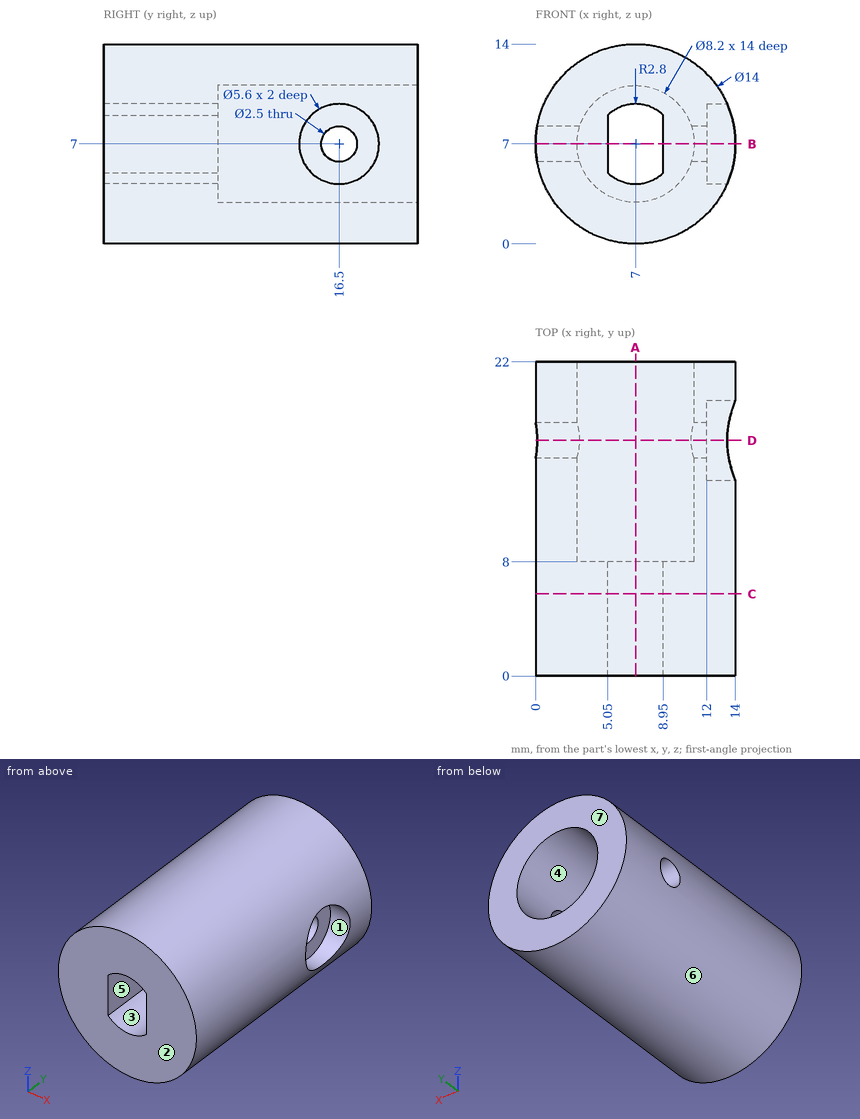
Drawing for the job (mm, zero at the part's lowest x, y, z). A direction names the side the tool comes from. Give positions to 0.01 mm unless a question says otherwise; leave off trailing zeros. Order: outer loops, then holes, each group sorted by start corner. A loop starts at its lowest first (then second) coordinate and runs counter-clockwise, first axis right, second up. Notation, with made-up numbers: (16, 34.25) - (41, 34.25) arc R21 cw to (41, 39.25) - close; hole circle Ø11 at (24.25, 49.25). An arc over 180 degrees is marked (long way). Use one line per item in the form item = value.
Item 1: Slice it at D-D on y = 16.5. Give the cut face in (x, z), and give its area (3 significant figures).
Solution:
outline = (0.11, 5.75) arc R7 ccw to (13.42, 4.2) - (12, 4.2) - (12, 5.75) - (10.9, 5.75) arc R4.1 cw to (3.1, 5.75) - close; (0.11, 8.25) - (3.1, 8.25) arc R4.1 cw to (10.9, 8.25) - (12, 8.25) - (12, 9.8) - (13.42, 9.8) arc R7 ccw to start
area = 81.3 mm2
Item 2: Pin check, flat tips, straight feed: pin 1 Ø3 at (y, z) = (16.5, 7) entering from -X; pin 2 Ø1.5 at (y, z) = (9, 2.5) entering from +X; pin 3 Ø5 at (y, z) = (16.5, 7) entering from +X; pin 4 Ø4 at (x, z) = (7.5, 6) entering from +Y. Stop position of each tip, or through.
Solution:
pin_1 = 0
pin_2 = 12.91
pin_3 = 12
pin_4 = 8
Item 3: Slice it at C-C on y = 5.75. Give the cut face in (x, z), and give its area (3 significant figures).
Solution:
outline = circle Ø14 at (7, 7); hole (5.05, 4.99) arc R2.8 ccw to (8.95, 4.99) - (8.95, 9.01) arc R2.8 ccw to (5.05, 9.01) - close
area = 134 mm2
Item 4: Which spindle directions (+Z, -Z, +X, -X, +Y, -Y) get a long thin tool onto all of the face, cutting with end or side? Do the marked faces 1, 2 and 3. Say none if no direction does.
Solution:
face_1 = +X
face_2 = +Z, -Z, +X, -X, -Y
face_3 = +Y, -Y
Item 5: Probe probe 1 along Y at (x, z) = (2.15, 7); probe 2 along Y at (x, z) = (12.5, 7); probe 3 along Y at (x, z) = (7.75, 10). List the from-to ranges inside material, lowest first. Write a range as from..to.
Solution:
probe_1 = 0..15.25, 17.75..22
probe_2 = 0..13.7, 19.3..22
probe_3 = 0..8
Item 6: Two-plate mould, pull along X, no slides. Class the marked faces 4, 5, 6 and 7: released by +X, released by -X, zero draft, split by the parting line, or undercut.
Solution:
face_4 = undercut
face_5 = undercut
face_6 = split by the parting line
face_7 = zero draft
Item 7: Slice it at A-A on x = 7. Give the cut face in (y, z).
Solution:
outline = (0, 0) - (22, 0) - (22, 2.9) - (8, 2.9) - (8, 4.2) - (0, 4.2) - close; (0, 9.8) - (8, 9.8) - (8, 11.1) - (22, 11.1) - (22, 14) - (0, 14) - close
Item 8: Slice it at B-B on z = 7. Give the cut face in (x, y), and give its area (3 significant figures).
Solution:
outline = (0, 0) - (5.05, 0) - (5.05, 8) - (2.9, 8) - (2.9, 15.25) - (0, 15.25) - close; (0, 17.75) - (2.9, 17.75) - (2.9, 22) - (0, 22) - close; (8.95, 0) - (14, 0) - (14, 13.7) - (12, 13.7) - (12, 15.25) - (11.1, 15.25) - (11.1, 8) - (8.95, 8) - close; (11.1, 17.75) - (12, 17.75) - (12, 19.3) - (14, 19.3) - (14, 22) - (11.1, 22) - close
area = 141 mm2
